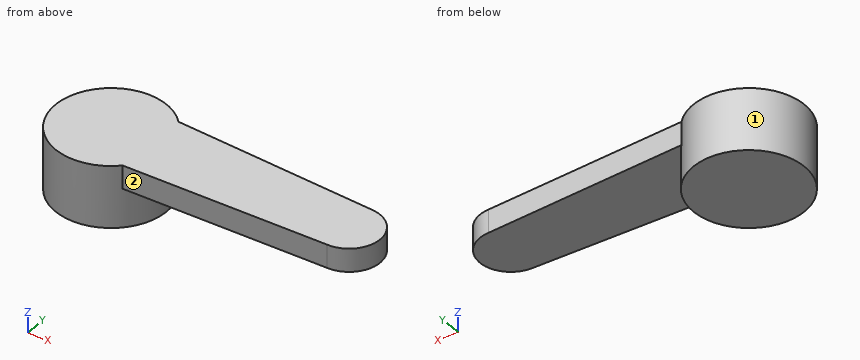
from build123d import *

# Parameters (mm, degrees)
SKETCH_1_R      = 3.6
EXTRUDE_1_DEPTH = 4
EXTRUDE_2_DEPTH = 1.5


with BuildPart() as part:
    # 草图1 → 凸台-拉伸1 (new body)
    with BuildSketch(Plane.XY):
        Circle(SKETCH_1_R)
    extrude(amount=EXTRUDE_1_DEPTH)

    # 草图2 → 凸台-拉伸2 (add)
    with BuildSketch(Plane.XY.offset(4)):
        with BuildLine():
            Line((2.590366769, 2.5), (15.6, 2))
            ThreePointArc((15.6, 2), (17.6, 0), (15.6, -2))
            Line((15.6, -2), (2.590366769, -2.5))
            Line((2.590366769, -2.5), (2.590366769, 2.5))
        make_face()
    extrude(amount=-EXTRUDE_2_DEPTH)


solid = part.part
Can you work these out from the model? Positions are in its coordinate system, mm. Face numbers are marked on the shaded views. A direction names the side the tool comes from. Give positions to 0.01 mm unless a question says otherwise; leave off trailing zeros. Loops run counter-clockwise (first coordinate to the right, second up) from the corner with the lowest first, then second, coordinate; pieces in that order, holes last. Notation, with made-up numbers: (-21.75, 80) -> (-2.75, 80) arc R16 cw to (-2.75, 109) -> close; hole circle Ø9 at (61, -39.5). An arc over 180 degrees is marked (long way). Return JSON: item names as keys, results as strings.
Q1. I want a section at A-A, the plane y = 0. List the corners of the cut face in (x, z) for me, then the cut area to 3 significant figures.
Checks:
{"outline": "(-3.6, 0) -> (3.6, 0) -> (3.6, 2.5) -> (17.6, 2.5) -> (17.6, 4) -> (-3.6, 4) -> close", "area": "49.8 mm2"}
Q2. On a 3-axis mill with a long thin cutter (end or side, diameter ignored), from which of +Z, -Z, +X, -X, +Y, -Y can I reach the whole of each face in a straight line? I mean the marked faces 1 and 2. Say none if no direction works.
Checks:
{"face 1": "-Z", "face 2": "+Z, -Z, +X, -Y"}
Q3. I want a section at C-C, the plane x = 12.25. List the corners of the cut face in (y, z) for me.
Checks:
{"outline": "(-2.13, 2.5) -> (2.13, 2.5) -> (2.13, 4) -> (-2.13, 4) -> close"}
Q4. For pin 1 Ø1.5 at (x, z) = (8, 2.5) entering from +Y; pin 2 Ø1.5 at (y, z) = (-1.5, 0.5) entering from +X, each with a flat end and sliding along its axis, tell me the tip position at first contact or that it passes through.
Checks:
{"pin 1": "stops at y = 2.32", "pin 2": "stops at x = 3.52"}
Q5. I need wall thicknesses on probe 1 along Z at (x, y) = (14, -1.5); probe 2 along X at (y, z) = (0, 0.95); probe 3 along X at (y, z) = (1, 3.3). Which ranges of each line are inside material? Lowest first, please.
Checks:
{"probe 1": "z = 2.5 to 4", "probe 2": "x = -3.6 to 3.6", "probe 3": "x = -3.46 to 17.33"}
Q6. I want a section at B-B, the plane z = 2.2. List the corners of the cut face in (x, y) for me, then the cut area to 3 significant figures.
Checks:
{"outline": "circle Ø7.2 at (0, 0)", "area": "40.7 mm2"}
Q7. I want a section at D-D, the plane y = -1.25. List the corners of the cut face in (x, z) for me.
Checks:
{"outline": "(-3.38, 0) -> (3.38, 0) -> (3.38, 2.5) -> (17.16, 2.5) -> (17.16, 4) -> (-3.38, 4) -> close"}
